Autodesk Inventor part; units mm, degrees
ref_plane "YZ Plane" through (0, 0, 0) normal (1, 0, 0) x (0, 1, 0)
ref_plane "XZ Plane" through (0, 0, 0) normal (0, 1, 0) x (-1, 0, 0)
ref_plane "XY Plane" through (0, 0, 0) normal (0, 0, 1) x (1, 0, 0)
sketch "Sketch1" plane through (0, 0, 0) normal (0, 0, 1) x (1, 0, 0)
  line L0 (-52.5, -12.7) -> (-52.5, 12.7)
  line L1 (43, 12.7) -> (52.5, 12.7)
  line L2 (52.5, 12.7) -> (52.5, -12.7)
  line L3 (52.5, -12.7) -> (-52.5, 12.7) construction
  line L4 (-52.5, -12.7) -> (-43, -12.7)
  line L5 (-43, 12.7) -> (-52.5, 12.7)
  line L6 (-52.5, 12.7) -> (-52.5, -12.7)
  line L7 (52.5, -12.7) -> (43.7955, -12.7)
  line L8 (43.7955, 12.7) -> (52.5, 12.7)
  line L9 (52.5, 12.7) -> (52.5, -12.7)
  circle A0 centre (-43.423, 7.694) radius 1.5
  circle A1 centre (-43.423, -7.706) radius 1.5
  line L10 (0, 19) -> (0, -21) construction
  line L11 (52.5, -12.7) -> (52.5, 12.7)
  line L12 (52.5, -12.7) -> (43, -12.7)
  line L13 (43, 12.7) -> (52.5, 12.7)
  line L14 (52.5, 12.7) -> (52.5, -12.7)
  circle A2 centre (43.423, 7.694) radius 1.5
  circle A3 centre (43.423, -7.706) radius 1.5
  line L15 (-43, 12.7) -> (0, 2.2981)
  line L16 (0, 2.2981) -> (0, 0)
  line L17 (-52.5, 0) -> (75, 0) construction
  line L18 (-43, -12.7) -> (0, -2.2981)
  line L19 (0, -2.2981) -> (0, 0)
  line L20 (43, 12.7) -> (0, 2.2981)
  line L21 (43, -12.7) -> (0, -2.2981)
  line L22 (-35.158, 8.5049) -> (-35.158, 0)
  line L23 (-35.158, 8.5049) -> (-9.4754, 2.2921)
  line L24 (-9.4754, 0) -> (-9.4754, 2.2921)
  line L25 (52.5, 12.7) -> (-52.5, -12.7) construction
  line L26 (-35.158, -8.5049) -> (-35.158, 0)
  line L27 (-9.4754, 0) -> (-9.4754, -2.2921)
  line L28 (-35.158, -8.5049) -> (-9.4754, -2.2921)
  line L29 (35.158, 8.5049) -> (35.158, 0)
  line L30 (35.158, 8.5049) -> (9.4754, 2.2921)
  line L31 (9.4754, 0) -> (9.4754, 2.2921)
  line L32 (35.158, -8.5049) -> (35.158, 0)
  line L33 (9.4754, 0) -> (9.4754, -2.2921)
  line L34 (35.158, -8.5049) -> (9.4754, -2.2921)
  line L35 (-43.423, 7.694) -> (43.423, 7.694) construction
  line L36 (-52.5, 12.7) -> (-43, 12.7)
  line L37 (0, 2.2981) -> (-43, 12.7)
  line L38 (0, 2.2981) -> (43, 12.7)
  line L39 (43, 12.7) -> (52.5, 12.7)
  line L40 (52.5, 12.7) -> (52.5, -12.7)
  line L41 (52.5, -12.7) -> (43, -12.7)
  line L42 (43, -12.7) -> (0, -2.2981)
  line L43 (0, -2.2981) -> (-43, -12.7)
  line L44 (-43, -12.7) -> (-52.5, -12.7)
  line L45 (-52.5, -12.7) -> (-52.5, 12.7)
  dimension "d0" = 105
  dimension "d1" = 15.4
  dimension "d4" = 9.077
  dimension "d5" = 3
  dimension "d6" = 3
extrude "Extrusion1" add sketch "Sketch1" along normal blind 1
properties part number "drill guide"
The model under review builds one solid part; all positions refer to its coordinate system, in mm. A direction names the side the tool comes from. Round coordinates to 2 decimals unless told otherwise and drop trailing zeros. Order: outer loops, then holes, each group sorted by start corner. A loop starts at its lowest first (then second) coordinate and runs counter-clockwise, first axis right, second up. Notation, with made-up numbers: M 47.25,49 L 90.25,49 A23 cw 90.25,63 Z; hole C 68,54 d4. An arc over 180 degrees is marked long. Use a Markdown table: item, result.
1) Tool access review of faces 1 (the face through (-21.8, -7.57, 0.49)), 2 (the face through (21.8, 7.57, 0.49)), 3 (the face through (-22.496, 5.442, 0.493)), 4 (the face through (-1, 0, 1)): name each direction out of +Z, -Z, +X, -X, +Y, -Y from which nothing blocks a thin tool from reaching the whole face with its end or side.
Report:
| item | result |
|---|---|
| face 1 | +Z, -Z, -Y |
| face 2 | +Z, -Z, +Y |
| face 3 | +Z, -Z |
| face 4 | +Z, +X, -X, +Y, -Y |
2) Draft analysis for pull direction X (two halves, no side actions). For faces 5 (the face through (22.496, 5.442, 0.493)), 6 (the face through (-1, 0, 0)), state which applies: released by +X, released by -X, zero draft, split by the parting line, or undercut.
Report:
| item | result |
|---|---|
| face 5 | undercut |
| face 6 | zero draft |
3) Insertion check: pin 1 (2.5 mm diameter, centred on x = -43.423, y = -7.706, fed in from +Z). The pin has a flat end and moves straight along its axis. Give the tip position at first contact, or say it passes through.
Report:
| item | result |
|---|---|
| pin 1 | through |
4) Consider section C-C (z = 0.8). Write out the cut boundary in (x, y), then the cut area to 3 significant figures.
Report:
| item | result |
|---|---|
| outline | M -52.5,-12.7 L -43,-12.7 L 0,-2.3 L 43,-12.7 L 52.5,-12.7 L 52.5,12.7 L 43,12.7 L 0,2.3 L -43,12.7 L -52.5,12.7 Z; hole C -43.42,-7.71 d3; hole C -43.42,7.69 d3; hole M -35.16,-8.5 L -9.48,-2.29 L -9.48,2.29 L -35.16,8.5 Z; hole M 9.48,-2.29 L 35.16,-8.5 L 35.16,8.5 L 9.48,2.29 Z; hole C 43.42,-7.71 d3; hole C 43.42,7.69 d3 |
| area | 1,190 mm^2 |
5) Wall thickness on line 1 along X through (y, z) = (1.5, 0.9); line 2 along Y through (x, z) = (11, 0.15); line 3 along Y through (x, z) = (-23, 0.4): over which ranges is each line inside the solid? List them lowest first. Write a range as [from, to].
Report:
| item | result |
|---|---|
| line 1 | [-52.5, -35.16], [-9.48, 9.48], [35.16, 52.5] |
| line 2 | [-4.96, -2.66], [2.66, 4.96] |
| line 3 | [-7.86, -5.56], [5.56, 7.86] |
6) Consider section D-D (x = -27). Write out the cut boundary in (y, z).
Report:
| item | result |
|---|---|
| outline | M -8.83,0 L -6.53,0 L -6.53,1 L -8.83,1 Z; M 6.53,0 L 8.83,0 L 8.83,1 L 6.53,1 Z |
7) Consider section B-B (y = 0.5). Write out the cut boundary in (x, z), then the cut area to 3 significant figures.
Report:
| item | result |
|---|---|
| outline | M -52.5,0 L -35.16,0 L -35.16,1 L -52.5,1 Z; M -9.48,0 L 9.48,0 L 9.48,1 L -9.48,1 Z; M 35.16,0 L 52.5,0 L 52.5,1 L 35.16,1 Z |
| area | 53.6 mm^2 |
8) Consider section A-A (y = -4.25). Write out the cut boundary in (x, z).
Report:
| item | result |
|---|---|
| outline | M -52.5,0 L -35.16,0 L -35.16,1 L -52.5,1 Z; M -17.57,0 L -8.07,0 L -8.07,1 L -17.57,1 Z; M 8.07,0 L 17.57,0 L 17.57,1 L 8.07,1 Z; M 35.16,0 L 52.5,0 L 52.5,1 L 35.16,1 Z |
